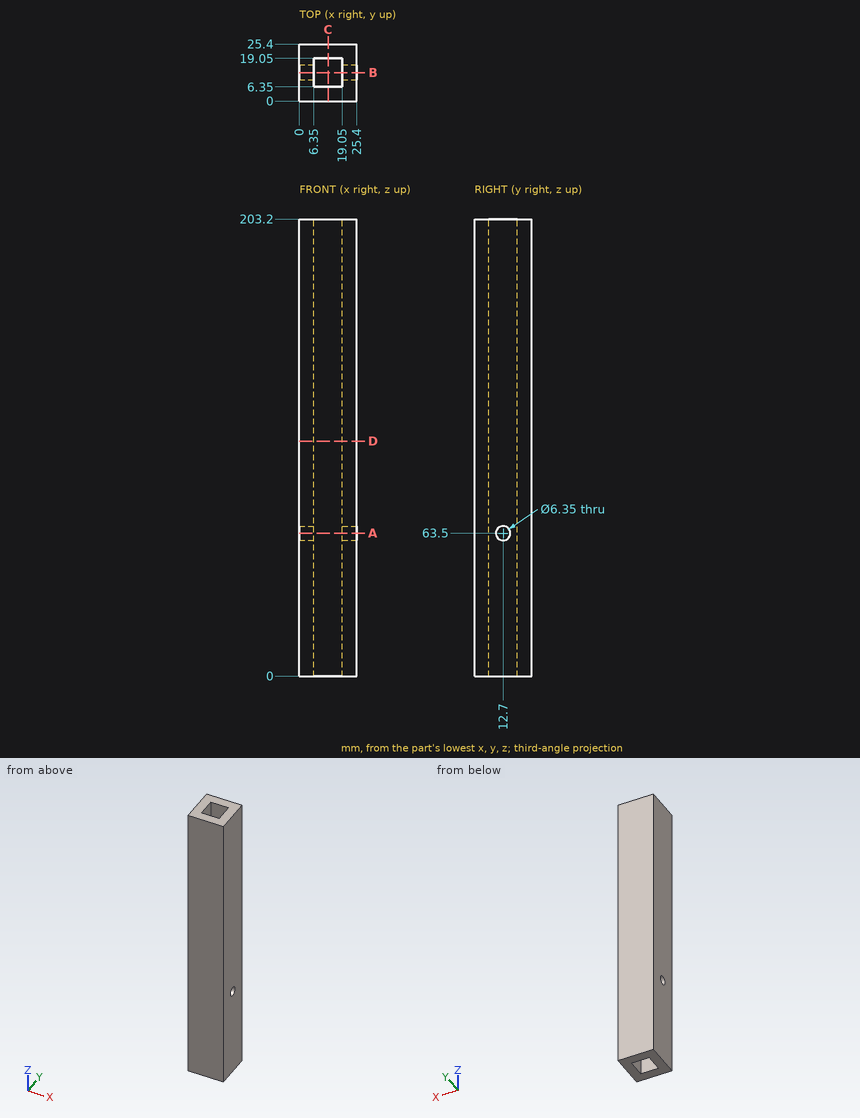
For this review, use the dimensioned drawing (mm, ordinates from the lowest corner) and the shaded views. Give positions to 0.01 mm unless a question says otherwise; leave off trailing zeros. Order: outer loops, then holes, each group sorted by start corner. A loop starts at its lowest first (then second) coordinate and runs counter-clockwise, first axis right, second up. Notation, with made-up numbers: (66.25, -22) -> (70.25, -22) arc R19 ccw to (70.25, -17) -> close; hole circle Ø10 at (55.25, 27.5). An arc over 180 degrees is marked (long way). Write item = value, one per line. Start each with the question number.
(1) Take a section at A-A (z = 63.5). Write out the cut boundary in (x, y) (3 decimals).
(2) Take a section at B-B (y = 12.7). Write out the cut boundary in (x, z) (3 decimals).
(3) For L1, parallel to Z at x = 5.25, y = 12.7 (3 decimals); L2, parallel to X at y = 14, z = 191.5; L3, parallel to Y at x = 6, z = 63, list the stretches that pass through material, from the lowest coordinate up. Write a range as from..to.
(4) Take a section at D-D (z = 104.5). Write out the cut boundary in (x, y), plus the area to 3 significant figures.
(5) Take a section at C-C (x = 12.75). Write out the cut boundary in (y, z), plus the area to 3 significant figures.
Returned:
q1.outline = (0, 0) -> (25.4, 0) -> (25.4, 9.525) -> (19.05, 9.525) -> (19.05, 6.35) -> (6.35, 6.35) -> (6.35, 9.525) -> (0, 9.525) -> close; (0, 15.875) -> (6.35, 15.875) -> (6.35, 19.05) -> (19.05, 19.05) -> (19.05, 15.875) -> (25.4, 15.875) -> (25.4, 25.4) -> (0, 25.4) -> close
q2.outline = (0, 0) -> (6.35, 0) -> (6.35, 60.325) -> (0, 60.325) -> close; (0, 66.675) -> (6.35, 66.675) -> (6.35, 203.2) -> (0, 203.2) -> close; (19.05, 0) -> (25.4, 0) -> (25.4, 60.325) -> (19.05, 60.325) -> close; (19.05, 66.675) -> (25.4, 66.675) -> (25.4, 203.2) -> (19.05, 203.2) -> close
q3.L1 = 0..60.325, 66.675..203.2
q3.L2 = 0..6.35, 19.05..25.4
q3.L3 = 0..9.56, 15.84..25.4
q4.outline = (0, 0) -> (25.4, 0) -> (25.4, 25.4) -> (0, 25.4) -> close; hole (6.35, 6.35) -> (19.05, 6.35) -> (19.05, 19.05) -> (6.35, 19.05) -> close
q4.area = 484 mm²
q5.outline = (0, 0) -> (6.35, 0) -> (6.35, 203.2) -> (0, 203.2) -> close; (19.05, 0) -> (25.4, 0) -> (25.4, 203.2) -> (19.05, 203.2) -> close
q5.area = 2,580 mm²
